For this review, take the finished solid that the model builds, in its own axes (mm). A direction names the side the tool comes from. Coordinates: 2 decimals unless noted, no trailing zeros. Loops run counter-clockwise (first coordinate to the right, second up) from the corner with the lowest first, then second, coordinate; pieces in that order, holes last. Notation, with made-up numbers: M -6.75,15 L 29.25,15 A8 cw 29.25,27 Z; hole C -40,3 d10. An arc over 180 degrees is marked long. Answer as a JSON object with one key per item and string values. Group by question number.
Item 1: Wall thickness on L1, parallel to X at y = 1.2, z = 11.5; L2, parallel to Y at x = 9, z = 0.65; L3, parallel to Y at x = 5.25, z = 14.75: over which ranges is each line inside the solid? List them lowest first. Write a range as from..to.
Item 2: Add section B-B (x = 9). State the section outline as (y, z) points, then the cut area to 3 significant figures.
Item 3: Insertion check: pin 1 (8 mm diameter, centred on x = 14, y = 15.5, fed in from +Z); pin 2 (7 mm diameter, centred on x = 7, z = 12.5, fed in from +Y). Each pin has a flat end and moves straight along its axis. Give the tip position at first contact, or say it passes through.
Item 4: Mouldability with a two-part tool opening along X and no side actions: class faces 1 (the face through (8.9, 8.5, 3)), 2 (the face through (0, 2.5, 5.6)), 3 (the face through (6.41, 1.52, 10.93)), 4 (the face through (18, 2.5, 5.6)) as +X half, -X half, draft (parallel to the pull), parting line (faces both ways), or undercut.
Item 5: Tool access review of faces 5 (the face through (8.9, 3, 8.5)), 6 (the face through (6.897, 9.888, 1.521)): name each direction out of +Z, -Z, +X, -X, +Y, -Y from which nothing blocks a thin tool from reaching the whole face with its end or side.
Item 6: Add section C-C (x = 5.25). State the section outline as (y, z) points, then the cut area to 3 significant figures.
Item 7: Add section D-D (z = 13). State the section outline as (x, y) points, then the cut area to 3 significant figures.
Item 8: Add section A-A (y = 11.5). State the section outline as (x, z) points, then the cut area to 3 significant figures.
from build123d import *

# Parameters (mm, degrees)
SKETCH1_W           = 18
SKETCH1_H           = 20
BOSS_EXTRUDE3_DEPTH = 3
SKETCH4_W           = 18
SKETCH4_H           = 3
BOSS_EXTRUDE4_DEPTH = 17
SKETCH5_R           = 2.65
CUT_EXTRUDE1_DEPTH  = 3
SKETCH6_R           = 2.65
CUT_EXTRUDE2_DEPTH  = 3
FILLET1_R           = 2.5


with BuildPart() as part:
    # Sketch1 → Boss-Extrude3 (new body)
    with BuildSketch(Plane(origin=(0, 0, 0), x_dir=(1, 0, 0), z_dir=(0, 1, 0))):
        with Locations((9, -10)):
            Rectangle(SKETCH1_W, SKETCH1_H)
    extrude(amount=BOSS_EXTRUDE3_DEPTH)

    # Sketch4 → Boss-Extrude4 (add)
    with BuildSketch(Plane(origin=(0, 3, 0), x_dir=(1, 0, 0), z_dir=(0, 1, 0))):
        with Locations((9, -1.5)):
            Rectangle(SKETCH4_W, SKETCH4_H)
    extrude(amount=BOSS_EXTRUDE4_DEPTH)

    # Sketch5 → Cut-Extrude1 (cut)
    with BuildSketch(Plane(origin=(0, 3, 0), x_dir=(1, 0, 0), z_dir=(0, 1, 0))):
        with Locations(Location((9, -11.5, 0), (0, 0, 270))):
            Circle(SKETCH5_R)
    extrude(amount=-CUT_EXTRUDE1_DEPTH, mode=Mode.SUBTRACT)

    # Sketch6 → Cut-Extrude2 (cut)
    with BuildSketch(Plane.XY.offset(3)):
        with Locations((9, 11.5)):
            Circle(SKETCH6_R)
    extrude(amount=-CUT_EXTRUDE2_DEPTH, mode=Mode.SUBTRACT)

    # Fillet1
    fillet1_edges = [part.edges().sort_by_distance(p)[0] for p in [
        (9, 20, 3),
        (9, 3, 20),
    ]]
    fillet(fillet1_edges, radius=FILLET1_R)


solid = part.part
From the geometry:
{
 "1": {"L1": "x = 0..6.35, 11.65..18", "L2": "y = 0..8.85, 14.15..20", "L3": "y = 0..3"},
 "2": {"outline": "M 0,0 L 8.85,0 L 8.85,3 L 3,3 L 3,8.85 L 0,8.85 Z; M 0,14.15 L 3,14.15 L 3,17.5 A2.5 ccw 0.5,20 L 0,20 Z; M 14.15,0 L 20,0 L 20,0.5 A2.5 ccw 17.5,3 L 14.15,3 Z", "area": "76.5 mm²"},
 "3": {"pin 1": "stops at z = 3", "pin 2": "stops at y = 3"},
 "4": {"face 1": "draft", "face 2": "-X half", "face 3": "undercut", "face 4": "+X half"},
 "5": {"face 5": "+Z, +X, -X, +Y", "face 6": "+Z, -Z"},
 "6": {"outline": "M 0,0 L 20,0 L 20,0.5 A2.5 ccw 17.5,3 L 3,3 L 3,17.5 A2.5 ccw 0.5,20 L 0,20 Z", "area": "108 mm²"},
 "7": {"outline": "M 0,0 L 6.82,0 L 6.82,3 L 0,3 Z; M 11.18,0 L 18,0 L 18,3 L 11.18,3 Z", "area": "40.9 mm²"},
 "8": {"outline": "M 0,0 L 6.35,0 L 6.35,3 L 0,3 Z; M 11.65,0 L 18,0 L 18,3 L 11.65,3 Z", "area": "38.1 mm²"}
}
